```python
from build123d import *

# Parameters (mm, degrees)
SKETCH1_R           = 77.4600051
BOSS_EXTRUDE1_DEPTH = 3.175
SKETCH24_R          = 22.1615
SKETCH24_R_2        = 2.54
SKETCH24_R_3        = 2.0193
CUT_EXTRUDE14_DEPTH = 110.590991442


with BuildPart() as part:
    # Sketch1 → Boss-Extrude1 (new body)
    with BuildSketch(Plane(origin=(0, 0, 0), x_dir=(1, 0, 0), z_dir=(0, 1, 0))):
        with Locations(Location((0, 0, 0), (0, 0, 270))):
            Circle(SKETCH1_R)
    extrude(amount=BOSS_EXTRUDE1_DEPTH)

    # Sketch24 → Cut-Extrude14 (cut, through all)
    with BuildSketch(Plane(origin=(0, 3.175, 0), x_dir=(1, 0, 0), z_dir=(0, 1, 0))):
        with Locations(Location((0, 0, 0), (0, 0, 270))):
            Circle(SKETCH24_R)
        with Locations(Location((-30.48, -30.48, 0), (0, 0, 270))):
            Circle(SKETCH24_R_2)
        with Locations(Location((0, -33.02, 0), (0, 0, 270))):
            Circle(SKETCH24_R_3)
        with Locations(Location((33.02, 0, 0), (0, 0, 270))):
            Circle(SKETCH24_R_3)
        with Locations(Location((0, 33.02, 0), (0, 0, 270))):
            Circle(SKETCH24_R_3)
        with Locations(Location((-33.02, 0, 0), (0, 0, 270))):
            Circle(SKETCH24_R_3)
        with Locations(Location((-25.4, 25.4, 0), (0, 0, 270))):
            Circle(SKETCH24_R_3)
    extrude(amount=-CUT_EXTRUDE14_DEPTH, mode=Mode.SUBTRACT)


solid = part.part
```
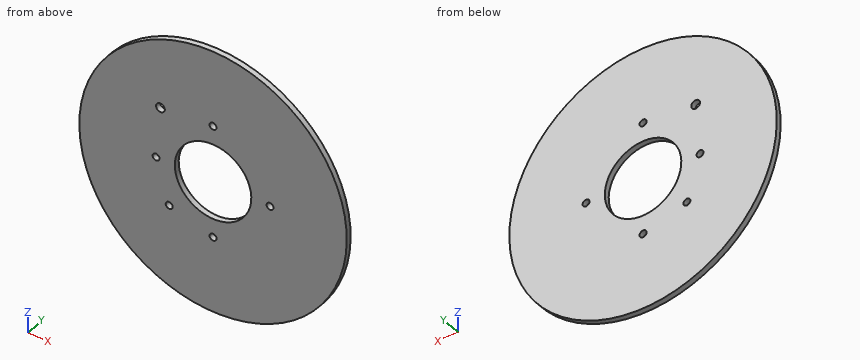
Design review of the part built by this model. Coordinates are the model's own, in mm. Coordinates: 2 decimals unless noted, no trailing zeros. Order: outer loops, then holes, each group sorted by start corner. A loop starts at its lowest first (then second) coordinate and runs counter-clockwise, first axis right, second up. Notation, with made-up numbers: M 78.25,-3.75 L 110.25,-3.75 A22 cw 110.25,22.25 Z; hole C 10,39 d11. An arc over 180 degrees is marked long. Answer as a JSON object with one key per item and string values. Group by question number.
1) Wall thickness on L1, parallel to X at y = 2.1, z = 32 (3 decimals); L2, parallel to Z at x = 0.5, y = 2.1; L3, parallel to Z at x = 20, y = 1.1: over which ranges is each line inside the solid? List them lowest first.
2) Add section A-A, the plane z = 0. Write out the cut boundary in (x, y) (1 decimal).
3) Add section C-C, the plane y = 1.7. Write out the cut boundary in (x, z), then the cut area to 3 significant figures.
4) Add section D-D, the plane z = -33.02. Write out the cut boundary in (x, y) (3 decimals).
5) Add section B-B, the plane x = 33.02. Write out the cut boundary in (y, z) (3 decimals).
6) For pin 1 (6.5 mm diameter, centred on x = 0, z = 33.02, fed in from +Y) (3 decimals); pin 2 (1.5 mm diameter, centred on x = 53, y = 0.5, fed in from -Z); pin 3 (3 mm diameter, centred on x = -25.4, z = -25.4, fed in from +Y); pin 4 (1.5 mm diameter, centred on y = 0.5, z = 10, fed in from +X), all flat-tipped, find the tip position at first contact; note any pin that passes through.
Computed values:
{
 "1": {"L1": "x = -70.541 to -32.515, -28.445 to -1.743, 1.743 to 70.541", "L2": "z = -77.46 to -34.98, -31.06 to -22.16, 22.16 to 31.06, 34.98 to 77.46", "L3": "z = -74.83 to -9.55, 9.55 to 74.83"},
 "2": {"outline": "M -77.5,0 L -35,0 L -35,3.2 L -77.5,3.2 Z; M -31,0 L -22.2,0 L -22.2,3.2 L -31,3.2 Z; M 22.2,0 L 31,0 L 31,3.2 L 22.2,3.2 Z; M 35,0 L 77.5,0 L 77.5,3.2 L 35,3.2 Z"},
 "3": {"outline": "C 0,0 d154.92; hole C -33.02,0 d4.04; hole C -30.48,30.48 d5.08; hole C -25.4,-25.4 d4.04; hole C 0,0 d44.32; hole C 0,-33.02 d4.04; hole C 0,33.02 d4.04; hole C 33.02,0 d4.04", "area": "17,200 mm^2"},
 "4": {"outline": "M -70.069,0 L -2.019,0 L -2.019,3.175 L -70.069,3.175 Z; M 2.019,0 L 70.069,0 L 70.069,3.175 L 2.019,3.175 Z"},
 "5": {"outline": "M 0,-70.069 L 3.175,-70.069 L 3.175,-2.019 L 0,-2.019 Z; M 0,2.019 L 3.175,2.019 L 3.175,70.069 L 0,70.069 Z"},
 "6": {"pin 1": "stops at y = 3.175", "pin 2": "stops at z = -57.18", "pin 3": "passes through", "pin 4": "stops at x = 76.91"}
}
